Autodesk Inventor part; units mm, degrees
ref_plane "YZ Plane" through (0, 0, 0) normal (1, 0, 0) x (0, 1, 0)
ref_plane "XZ Plane" through (0, 0, 0) normal (0, 1, 0) x (-1, 0, 0)
ref_plane "XY Plane" through (0, 0, 0) normal (0, 0, 1) x (1, 0, 0)
sketch "Эскиз1" plane through (0, 0, 0) normal (0, 0, 1) x (1, 0, 0)
  circle A0 centre (0, 0) radius 1.5
  circle A1 centre (0, 0) radius 2.75
  dimension "d0" = 5.5
  dimension "d1" = 3
extrude "Выдавливание1" add sketch "Эскиз1" along normal blind 6 contours A0
extrude "Выдавливание2" add sketch "Эскиз1" against normal blind 1.5 contours A0 | A1
thread "Резьба1"
sketch "Эскиз2" plane through (0, 0, -1.5) normal (0, 0, -1) x (-1, 0, 0)
  line L0 (0, 1.1547) -> (1, 0.5774)
  line L1 (1, 0.5774) -> (1, -0.5774)
  line L2 (1, -0.5774) -> (0, -1.1547)
  line L3 (0, -1.1547) -> (-1, -0.5774)
  line L4 (-1, -0.5774) -> (-1, 0.5774)
  line L5 (-1, 0.5774) -> (0, 1.1547)
  point P0 (0, 0)
  point P1 (0, 0)
  dimension "d8" = 2
extrude "Выдавливание3" cut sketch "Эскиз2" against normal blind 1
fillet "Сопряжение1" radius 1 1 edges at (-2.75, 0, -1.5)
properties part number "Болт М3 6 мм"
Design review of the part built by this model. Coordinates are the model's own, in mm. A direction names the side the tool comes from. Give positions to 0.01 mm unless a question says otherwise; leave off trailing zeros. Loops run counter-clockwise (first coordinate to the right, second up) from the corner with the lowest first, then second, coordinate; pieces in that order, holes last. Notation, with made-up numbers: (-23.5, 35) -> (-13.5, 35) arc R27 cw to (-13.5, 70) -> close; hole circle Ø10 at (22, 35). An arc over 180 degrees is marked (long way). One line per item, written item: value.
Q1. We need section C-C on z = 5.25. Give the boundary of the cut face in (x, y), and give its area (3 significant figures).
Numbers:
outline: circle Ø3 at (0, 0)
area: 7.07 mm^2
Q2. For pin 1 Ø3 at (x, z) = (2, 4.5) entering from -Y; pin 2 Ø1 at (y, z) = (-1, 3.5) entering from -X; pin 3 Ø1.1 at (y, z) = (0, -1) entering from -X; pin 4 Ø0.8 at (y, z) = (0, -1) entering from +X (3 decimals), all flat-tipped, find the tip position at first contact; note any pin that passes through.
Numbers:
pin 1: stops at y = -1.41
pin 2: stops at x = -1.41
pin 3: stops at x = -2.75
pin 4: stops at x = 2.745
Q3. We need section A-A on y = 0. Give the boundary of the cut face in (x, z).
Numbers:
outline: (-2.75, -0.5) arc R1 ccw to (-1.75, -1.5) -> (-1, -1.5) -> (-1, -0.5) -> (1, -0.5) -> (1, -1.5) -> (1.75, -1.5) arc R1 ccw to (2.75, -0.5) -> (2.75, 0) -> (1.5, 0) -> (1.5, 6) -> (-1.5, 6) -> (-1.5, 0) -> (-2.75, 0) -> close
Q4. Machinability: for faces 4 (the flat face through (1, -1, -1.5)), 5 (the cylindrical face through (-1.5, -0.07, 2.96)), 6 (the flat face through (0.49, -0.87, -1.01)), which of the approach directions +Z, -Z, +X, -X, +Y, -Y give a long, thin tool a straight path to every point of the face, cutting with its end or side? Answer none if there is none.
Numbers:
face 4: -Z, +X, -X, +Y, -Y
face 5: +Z
face 6: -Z
Q5. Draft analysis for pull direction X (two halves, no side actions). For faces 1 (the flat face through (-0.49, 0.87, -1.01)), 2 (the flat face through (1.2, -1.2, 0)), 3 (the cylindrical face through (-0.596, -2.685, -0.246)), state which applies: pulls with the +X half, pulls with the -X half, needs draft (parallel to the pull), parting line crosses it, or undercut.
Numbers:
face 1: undercut
face 2: needs draft
face 3: parting line crosses it
Q6. We need section B-B on z = -0.75. Give the boundary of the cut face in (x, y), and give its area (3 significant figures).
Numbers:
outline: circle Ø5.44 at (0, 0); hole (-1, -0.58) -> (0, -1.15) -> (1, -0.58) -> (1, 0.58) -> (0, 1.15) -> (-1, 0.58) -> close
area: 19.7 mm^2
Q7. For L1, parallel to Z at x = 0.25, y = 1.6; L2, parallel to Y at x = -0.05, z = 2.75; L3, parallel to Z at x = -0.2, y = -0.5, list the stretches that pass through material, from the lowest coordinate up.
Numbers:
L1: z = -1.5 to 0
L2: y = -1.5 to 1.5
L3: z = -0.5 to 6
